The model under review builds one solid part; all positions refer to its coordinate system, in mm. Face numbers are marked on the shaded views. A direction names the side the tool comes from. Coordinates: 2 decimals unless noted, no trailing zeros. Order: outer loops, then holes, each group sorted by start corner. A loop starts at its lowest first (then second) coordinate and runs counter-clockwise, first axis right, second up. Notation, with made-up numbers: (86, 47) -> (119, 47) arc R30 cw to (119, 84) -> close; hole circle Ø10 at (-27.75, 30.25). An arc over 180 degrees is marked (long way). Use one line per item in the form item = value.
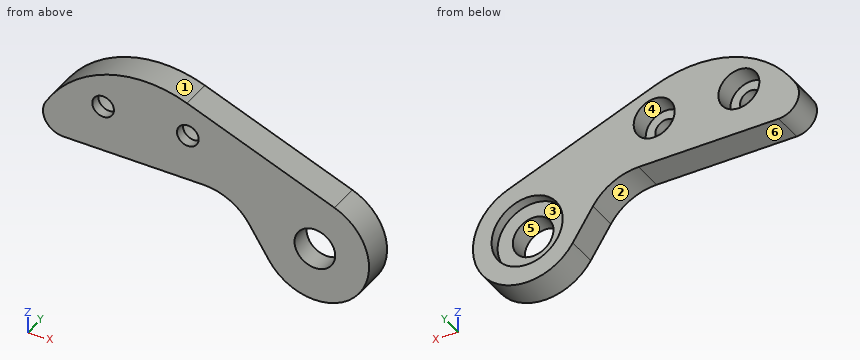
from build123d import *

# Parameters (mm, degrees)
EXTRUDE_1_DEPTH             = 4.5
HOLE_WIZARD_M31_D           = 3.2
HOLE_WIZARD_M31_CBORE_D     = 6.05
HOLE_WIZARD_M31_CBORE_DEPTH = 3
HOLE_WIZARD_1_D             = 6
HOLE_WIZARD_1_CBORE_D       = 10.5
HOLE_WIZARD_1_CBORE_DEPTH   = 1.5
FILLET_1_R                  = 8


with BuildPart() as part:
    # Эскиз1 → Бобышка-Вытянуть1 (new body)
    with BuildSketch(Plane.XZ):
        with BuildLine():
            Line((-12.124355653, 4), (12.936430666, 4))
            Line((12.936430666, 4), (18.263831879, -4.315557791))
            ThreePointArc((18.263831879, -4.315557791), (31.197157109, -5.059174218), (27.88, 7.463618425))
            Line((27.88, 7.463618425), (6.12, 15.860189154))
            ThreePointArc((6.12, 15.860189154), (-5.660702659, 16.029861054), (-14.722431864, 8.5))
            ThreePointArc((-14.722431864, 8.5), (-14.722431864, 5.5), (-12.124355653, 4))
        make_face()
    extrude(amount=-EXTRUDE_1_DEPTH)

    # Цековка для винта с заклепочной головкой M31 (through all)
    with Locations(Plane(origin=(0, 4.5, 0), x_dir=(1, 0, 0), z_dir=(0, 1, 0))):
        with Locations((-6.25, -10.825317547), (6.25, -10.825317547)):
            CounterBoreHole(HOLE_WIZARD_M31_D / 2, HOLE_WIZARD_M31_CBORE_D / 2, HOLE_WIZARD_M31_CBORE_DEPTH)

    # Отверстие1 (through all)
    with Locations(Plane(origin=(0, 4.5, 0), x_dir=(1, 0, 0), z_dir=(0, 1, 0))):
        with Locations((25, 0)):
            CounterBoreHole(HOLE_WIZARD_1_D / 2, HOLE_WIZARD_1_CBORE_D / 2, HOLE_WIZARD_1_CBORE_DEPTH)

    # Скругление1
    fillet_1_edges = [part.edges().sort_by_distance(p)[0] for p in [
        (12.936430666, 2.25, 4),
    ]]
    fillet(fillet_1_edges, radius=FILLET_1_R)


solid = part.part
Item 1: We need section C-C (z = -1.5). Write out the cut boundary in (x, y).
Results found:
outline = (16.46, 0) -> (22.4, 0) -> (22.4, 3) -> (19.97, 3) -> (19.97, 4.5) -> (16.46, 4.5) -> close; (27.6, 0) -> (32.86, 0) -> (32.86, 4.5) -> (30.03, 4.5) -> (30.03, 3) -> (27.6, 3) -> close
Item 2: We need section D-D (z = 4.5). Write out the cut boundary in (x, y), plus the area to 3 significant figures.
Results found:
outline = (-13.78, 0) -> (31.61, 0) -> (31.61, 4.5) -> (27.7, 4.5) -> (27.7, 3) -> (22.3, 3) -> (22.3, 4.5) -> (-13.78, 4.5) -> close
area = 196 mm²
Item 3: Draft analysis for pull direction X (two halves, no side actions). For the marked faces 1, 2 and 3, state which applies: released by +X, released by -X, zero draft, split by the parting line, or undercut.
Results found:
face_1 = split by the parting line
face_2 = released by -X
face_3 = undercut
Item 4: Clearance check with flat-ended pins moving along their axes: pin 1 (3 mm diameter, centred on x = 6.25, z = 10.83, fed in from -Y); pin 2 (1 mm diameter, centred on y = 2, z = -5, fed in from +X); pin 3 (3 mm diameter, centred on x = -7.5, z = 11, fed in from +Y); pin 4 (2 mm diameter, centred on x = 21.5, z = 2, fed in from +Y). State where each tip first meets the part, or that it passes through.
Results found:
pin_1 = through
pin_2 = 31.61
pin_3 = 1.5
pin_4 = 3
Item 5: We need section B-B (y = 3.7). Write out the cut boundary in (x, z) (3 decimals).
Results found:
outline = (-14.722, 8.5) arc R3 ccw to (-12.124, 4) -> (8.561, 4) arc R8 cw to (15.297, 0.316) -> (18.264, -4.316) arc R8 ccw (long way) to (27.88, 7.464) -> (6.12, 15.86) arc R17 ccw to start; hole circle Ø6.05 at (-6.25, 10.825); hole circle Ø6.05 at (6.25, 10.825); hole circle Ø10.5 at (25, 0)
Item 6: Tool access review of the marked faces 4, 5 and 6: name each direction out of +Z, -Z, +X, -X, +Y, -Y from which nothing blocks a thin tool from reaching the whole face with its end or side.
Results found:
face_4 = +Y
face_5 = +Y, -Y
face_6 = -Z, -X, +Y, -Y
Item 7: We need section A-A (x = 27). Write out the cut boundary in (y, z), plus the area to 3 significant figures.
Results found:
outline = (0, -7.75) -> (4.5, -7.75) -> (4.5, -4.85) -> (3, -4.85) -> (3, -2.24) -> (0, -2.24) -> close; (0, 2.24) -> (3, 2.24) -> (3, 4.85) -> (4.5, 4.85) -> (4.5, 7.8) -> (0, 7.8) -> close
area = 42.0 mm²
Item 8: To check wall thickness, follow L1, parallel to Z at x = 6.25, y = 1.25; L2, parallel to Z at x = 0, y = 2.65; L3, parallel to Z at x = 25, y = 1.5. State the ranges of each line that lie inside material, in increasing order. Write a range as from..to.
Results found:
L1 = 4..9.23, 12.43..15.81
L2 = 4..17
L3 = -8..-3, 3..8.57
